```python
from build123d import *

# Parameters (mm, degrees)
CUT_EXTRUDE1_DEPTH = 5


with BuildPart() as part:
    # Sketch1 → Revolve1 (revolve)
    with BuildSketch(Plane.XY):
        with BuildLine():
            Line((12.5, 0), (0, 0))
            Line((0, 0), (0, 12.5))
            ThreePointArc((0, 12.5), (8.838834765, 8.838834765), (12.5, 0))
        make_face()
    revolve(axis=Axis((0, 0, 0), (0, 1, 0)))

    # Sketch2 → Cut-Extrude1 (cut)
    with BuildSketch(Plane(origin=(0, 0, 0), x_dir=(1, 0, 0), z_dir=(0, 1, 0))):
        Polygon((0, 9), (2.556172718, 3.518269915), (8.559508647, 2.781152949), (4.13597434, -1.343859526), (5.290067271, -7.281152949), (0, -4.348820778), (-5.290067271, -7.281152949), (-4.13597434, -1.343859526), (-8.559508647, 2.781152949), (-2.556172718, 3.518269915), align=None)
    extrude(amount=CUT_EXTRUDE1_DEPTH, mode=Mode.SUBTRACT)


solid = part.part
```
Work out the finished part from the listing and answer in its coordinate system (mm). Coordinates: 2 decimals unless noted, no trailing zeros. Loops run counter-clockwise (first coordinate to the right, second up) from the corner with the lowest first, then second, coordinate; pieces in that order, holes last. Notation, with made-up numbers: (73.25, 60) -> (87.25, 60) arc R12 cw to (87.25, 65) -> close; hole circle Ø9 at (-3, -18). An arc over 180 degrees is marked (long way). Answer as CSV lines item,"result".
Q1. The part is cut by section C-C on x = 6. Write down the section's boundary in (y, z).
Findings:
outline,"(0, -10.97) arc R10.97 ccw to (0, 10.97) -> (0, -0.39) -> (5, -0.39) -> (5, -3.1) -> (0, -3.1) -> close"
Q2. Each of these flat-tipped pins is pushed along its axis until it touches: pin 1 (1.5 mm diameter, centred on x = -3, z = -8, fed in from +Y); pin 2 (1.5 mm diameter, centred on x = -1.5, y = 4, fed in from +Z); pin 3 (3 mm diameter, centred on x = 5, y = 6, fed in from -Z). Where does it stop, or does it pass through?
Findings:
pin 1,"stops at y = 9.77"
pin 2,"stops at z = 11.99"
pin 3,"stops at z = -10.79"
Q3. The part is cut by section D-D on y = 1.75. Write down the section's boundary in (x, z).
Findings:
outline,"circle Ø24.75 at (0, 0); hole (-8.56, -2.78) -> (-2.56, -3.52) -> (0, -9) -> (2.56, -3.52) -> (8.56, -2.78) -> (4.14, 1.34) -> (5.29, 7.28) -> (0, 4.35) -> (-5.29, 7.28) -> (-4.14, 1.34) -> close"
Q4. The part is cut by section A-A on y = 3.5. Write down the section's boundary in (x, z).
Findings:
outline,"circle Ø24 at (0, 0); hole (-8.56, -2.78) -> (-2.56, -3.52) -> (0, -9) -> (2.56, -3.52) -> (8.56, -2.78) -> (4.14, 1.34) -> (5.29, 7.28) -> (0, 4.35) -> (-5.29, 7.28) -> (-4.14, 1.34) -> close"
Q5. Find the intervals of material crossed by probe 1 along Z at (x, y) = (-6.75, 4); probe 2 along Z at (x, y) = (2.75, 2.75); probe 3 along Y at (x, z) = (-2.75, 8), in increasing order.
Findings:
probe 1,"z = -9.73 to -3, -1.09 to 9.73"
probe 2,"z = -11.88 to -3.49, 5.87 to 11.88"
probe 3,"y = 0 to 9.2"
Q6. For a pull along Z with two mould halves and no side action, classify faces 1 (the face through (4.705, 2.465, 4.271)), 2 (the face through (0, 0, 5)) as +Z half, -Z half, draft (parallel to the pull), parting line (faces both ways), or undercut.
Findings:
face 1,"undercut"
face 2,"draft"
Q7. The part is cut by section B-B on z = 3.75. Write down the section's boundary in (x, y), and give its area (3 significant figures).
Findings:
outline,"(-11.92, 0) -> (-4.6, 0) -> (-4.6, 5) -> (4.6, 5) -> (4.6, 0) -> (11.92, 0) arc R11.92 ccw to start"
area,"177 mm²"
